```python
from build123d import *

# Parameters (mm, degrees)
F0_W     = 42.8
F0_H     = 32.4
F0_W_2   = 22.8
F0_H_2   = 12.4
F1_DEPTH = 24
F2_W     = 42.8
F2_H     = 32.4
F3_DEPTH = 5
F4_W     = 5
F4_H     = 10
F5_DEPTH = 25.4


with BuildPart() as f1:
    # F0 (on Top) → F1 (new body)
    with BuildSketch(Plane.XY):
        Rectangle(F0_W, F0_H)
        Rectangle(F0_W_2, F0_H_2, mode=Mode.SUBTRACT)
    extrude(amount=F1_DEPTH)

    # F2 (on face) → F3 (join)
    with BuildSketch(Plane(origin=(0, 0, 0), x_dir=(1, 0, 0), z_dir=(0, 0, -1))):
        Rectangle(F2_W, F2_H)
    extrude(amount=F3_DEPTH)

    # F4 (on face) → F5 (cut)
    with BuildSketch(Plane(origin=(-21.4, 0, 0), x_dir=(0, -1, 0), z_dir=(-1, 0, 0))):
        with Locations((0.08081, 10.283196)):
            Rectangle(F4_W, F4_H)
    extrude(amount=-F5_DEPTH, mode=Mode.SUBTRACT)


solid = f1.part
```
CAD build for the part. Positions are in the model's coordinates, mm. A direction names the side the tool comes from. Round coordinates to 2 decimals unless told otherwise and drop trailing zeros. Order: outer loops, then holes, each group sorted by start corner. A loop starts at its lowest first (then second) coordinate and runs counter-clockwise, first axis right, second up. Notation, with made-up numbers: (-33.5, 47) -> (-6.5, 47) arc R13 ccw to (-6.5, 64) -> close; hole circle Ø8 at (32.25, 59). An arc over 180 degrees is marked (long way). Write item = value, one per line.
(1) Cut at C-C (z = 11.5). Write the cut outline in (x, y), plus the area to 3 significant figures.
Answers follow:
outline = (-21.4, -16.2) -> (21.4, -16.2) -> (21.4, 16.2) -> (-21.4, 16.2) -> (-21.4, 2.42) -> (-11.4, 2.42) -> (-11.4, 6.2) -> (11.4, 6.2) -> (11.4, -6.2) -> (-11.4, -6.2) -> (-11.4, -2.58) -> (-21.4, -2.58) -> close
area = 1,050 mm²
(2) Cut at D-D (x = 9.5). Write the cut outline in (y, z), plus the area to 3 significant figures.
Answers follow:
outline = (-16.2, -5) -> (16.2, -5) -> (16.2, 24) -> (6.2, 24) -> (6.2, 0) -> (-6.2, 0) -> (-6.2, 24) -> (-16.2, 24) -> close
area = 642 mm²
(3) Drill centre lines: L1, parallel to X at y = -4, z = 6.25; L2, parallel to Y at x = -9, z = 19; L3, parallel to Z at x = -11.5, y = 0.5. Where is each one in solid material? Low to high.
Answers follow:
L1 = -21.4 to -11.4, 11.4 to 21.4
L2 = -16.2 to -6.2, 6.2 to 16.2
L3 = -5 to 5.28, 15.28 to 24
(4) Flat gauge pin, fed straight in: P1, Ø3.5, axis at x = -3, y = -1, coming from the +Z side. Where does the tip first touch, or does it go through?
Answers follow:
P1 = 0
(5) Cut at A-A (z = 21.25). Write the cut outline in (x, y).
Answers follow:
outline = (-21.4, -16.2) -> (21.4, -16.2) -> (21.4, 16.2) -> (-21.4, 16.2) -> close; hole (-11.4, -6.2) -> (11.4, -6.2) -> (11.4, 6.2) -> (-11.4, 6.2) -> close
(6) 3-axis set-ups, long thin cutter, end or side, ignore diameter. For faces 4 (the flat face through (0, -6.2, 12)), 5 (the flat face through (-16, 0, 15.283)), 6 (the flat face through (0, -16.2, 10)): which of +Z, -Z, +X, -X, +Y, -Y reach the whole face in a straight line?
Answers follow:
face_4 = +Z
face_5 = -X
face_6 = +Z, -Z, +X, -X, -Y
(7) Cut at B-B (x = -17.5). Write the cut outline in (y, z).
Answers follow:
outline = (-16.2, -5) -> (16.2, -5) -> (16.2, 24) -> (-16.2, 24) -> close; hole (-2.58, 5.28) -> (2.42, 5.28) -> (2.42, 15.28) -> (-2.58, 15.28) -> close
(8) Pull direction Y, two halves, no side cores. Call faces 1 (the flat face through (0, 16.2, 10)), 2 (the flat face through (-21.4, 4, 10)), 3 (the flat face through (-16, 2.419, 10)): +Y half, -Y half, draft (parallel to the pull), parting line (faces both ways), or undercut.
Answers follow:
face_1 = +Y half
face_2 = draft
face_3 = undercut
